```python
from build123d import *

# Parameters (mm, degrees)
SKETCH1_W           = 50.8
SKETCH1_H           = 76.2
BOSS_EXTRUDE1_DEPTH = 1.6
SKETCH3_W           = 22.86
SKETCH3_H           = 5.08
BOSS_EXTRUDE2_DEPTH = 0.1
SKETCH6_W           = 28.557161976
SKETCH6_H           = 42.013432375
BOSS_EXTRUDE3_DEPTH = 2


with BuildPart() as part:
    # Sketch1 → Boss-Extrude1 (new body)
    with BuildSketch(Plane.XY):
        Rectangle(SKETCH1_W, SKETCH1_H)
    extrude(amount=BOSS_EXTRUDE1_DEPTH)

    # Sketch3 → Boss-Extrude2 (add)
    with BuildSketch(Plane.XY.offset(1.6)):
        with Locations((0, 30.56)):
            Rectangle(SKETCH3_W, SKETCH3_H)
    extrude(amount=BOSS_EXTRUDE2_DEPTH)

    # Sketch6 → Boss-Extrude3 (add)
    with BuildSketch(Plane(origin=(0, 0, 0), x_dir=(-1, 0, 0), z_dir=(0, 0, -1))):
        with Locations((0, 1.728458928)):
            Rectangle(SKETCH6_W, SKETCH6_H)
    extrude(amount=BOSS_EXTRUDE3_DEPTH)


solid = part.part
```
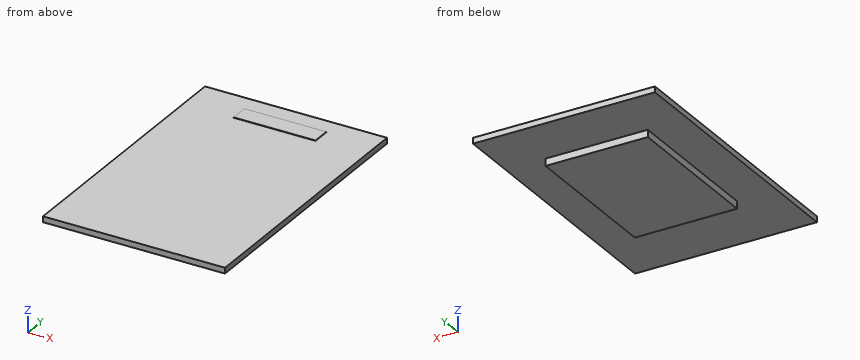
Here's how the part is built. I have some questions about the finished solid (model axes, mm). Coordinates: 2 decimals unless noted, no trailing zeros. Order: outer loops, then holes, each group sorted by start corner. A loop starts at its lowest first (then second) coordinate and runs counter-clockwise, first axis right, second up. Notation, with made-up numbers: (50.5, 55) -> (91.5, 55) arc R20 cw to (91.5, 93) -> close; hole circle Ø8 at (69.25, -23.5). An arc over 180 degrees is marked (long way). Return JSON: item names as keys, results as strings.
1) If I drill on probe 1 along Z at (x, y) = (-22.5, -21.5); probe 2 along Y at (x, z) = (5.5, -0.15); probe 3 along X at (y, z) = (-3.5, -0.55), over which ranges is the centre line in solid material (lowest first)?
Conclusion:
{"probe 1": "z = 0 to 1.6", "probe 2": "y = -19.28 to 22.74", "probe 3": "x = -14.28 to 14.28"}
2) If we section it at B-B on y = -5: List the corners of the cut face in (x, z) for me, plus the area to 3 significant figures.
Conclusion:
{"outline": "(-25.4, 0) -> (-14.28, 0) -> (-14.28, -2) -> (14.28, -2) -> (14.28, 0) -> (25.4, 0) -> (25.4, 1.6) -> (-25.4, 1.6) -> close", "area": "138 mm²"}
3) If we section it at D-D on y = 30.5: List the corners of the cut face in (x, z) for me.
Conclusion:
{"outline": "(-25.4, 0) -> (25.4, 0) -> (25.4, 1.6) -> (11.43, 1.6) -> (11.43, 1.7) -> (-11.43, 1.7) -> (-11.43, 1.6) -> (-25.4, 1.6) -> close"}
4) I'm going to push flat-ended pins straight in: P1, Ø5, axis at x = -0.5, y = 5.5, coming from the +Z side; P2, Ø0.6, axis at x = -7, z = -1, coming from the +Y side; P3, Ø0.6, axis at y = 2, z = -1.5, coming from the -X side. Where does each tip first touch, or does it pass through?
Conclusion:
{"P1": "stops at z = 1.6", "P2": "stops at y = 22.74", "P3": "stops at x = -14.28"}
5) If we section it at A-A on x = 7: List the corners of the cut face in (y, z) for me.
Conclusion:
{"outline": "(-38.1, 0) -> (-19.28, 0) -> (-19.28, -2) -> (22.74, -2) -> (22.74, 0) -> (38.1, 0) -> (38.1, 1.6) -> (33.1, 1.6) -> (33.1, 1.7) -> (28.02, 1.7) -> (28.02, 1.6) -> (-38.1, 1.6) -> close"}
6) If we section it at C-C on z = -0.65: List the corners of the cut face in (x, y) for me.
Conclusion:
{"outline": "(-14.28, -19.28) -> (14.28, -19.28) -> (14.28, 22.74) -> (-14.28, 22.74) -> close"}
